Read the model definition and answer for the solid it produces. Units are mm, in the model's axes. A direction names the side the tool comes from. Give positions to 0.01 mm unless a question says otherwise; leave off trailing zeros. Order: outer loops, then holes, each group sorted by start corner. A loop starts at its lowest first (then second) coordinate and runs counter-clockwise, first axis right, second up. Notation, with made-up numbers: (71, 73) - (92, 73) arc R18 cw to (92, 96) - close; hole circle Ø4 at (27, -3). An arc over 180 degrees is marked (long way). Return JSON: item names as keys, results as strings.
Autodesk Inventor part; units mm, degrees
ref_plane "YZ Plane" through (0, 0, 0) normal (1, 0, 0) x (0, 1, 0)
ref_plane "XZ Plane" through (0, 0, 0) normal (0, 1, 0) x (-1, 0, 0)
ref_plane "XY Plane" through (0, 0, 0) normal (0, 0, 1) x (1, 0, 0)
sketch "Sketch1" plane through (0, 0, 0) normal (1, 0, 0) x (0, 1, 0)
  line L0 (0, 0) -> (241.3, 0)
  line L1 (241.3, 0) -> (241.3, -25.4)
  line L2 (241.3, -25.4) -> (0, -25.4)
  line L3 (0, -25.4) -> (0, 0)
  line L4 (6.3489, -9.0357) -> (12.6978, -5.3677)
  line L5 (12.6978, -5.3677) -> (19.0489, -9.0319)
  line L6 (19.0489, -9.0319) -> (19.0511, -16.3643)
  line L7 (19.0511, -16.3643) -> (12.7022, -20.0323)
  line L8 (12.7022, -20.0323) -> (6.3511, -16.3681)
  line L9 (6.3511, -16.3681) -> (6.3489, -9.0357)
  point P0 (12.7, -12.7)
  dimension "d0" = 241.3
  dimension "d1" = 25.4
  dimension "d3" = 12.7
  dimension "d4" = 12.7
extrude "Extrusion1" add sketch "Sketch1" along normal blind 25.4
sketch "Sketch2" plane through (0, 241.3, 0) normal (0, 1, 0) x (1, 0, 0)
  line L0 (0, 25.4) -> (25.4, 25.4)
  line L1 (0, 0) -> (25.4, 0)
  line L2 (25.4, 0) -> (25.4, 25.4)
  line L3 (25.4, 25.4) -> (0, 25.4)
  line L4 (0, 25.4) -> (0, 0)
  line L5 (22.225, 3.175) -> (3.175, 3.175)
  line L6 (3.175, 3.175) -> (3.175, 22.225)
  line L7 (3.175, 22.225) -> (22.225, 22.225)
  line L8 (22.225, 22.225) -> (22.225, 3.175)
  dimension "d7" = 3.175
extrude "Extrusion2" cut sketch "Sketch2" against normal blind 228.6 contours L5 L6 L7 L8
sketch "Sketch3" plane through (25.4, 0, 0) normal (1, 0, 0) x (0, 0, -1)
  line L0 (0, 241.3) -> (0, 190.5)
  line L1 (0, 0) -> (0, 241.3)
  line L2 (0, 241.3) -> (-3.175, 241.3)
  line L3 (-3.175, 241.3) -> (-3.175, 190.5)
  line L4 (-3.175, 190.5) -> (0, 190.5)
  line L5 (0, 190.5) -> (0, 241.3)
  arc A0 (-3.175, 241.3) -> (-46.143, 196.9282) centre (-8.4506, 203.4185) ccw
  line L6 (-3.175, 241.3) -> (-3.175, 238.125)
  arc A1 (-3.175, 238.125) -> (-42.9327, 197.9157) centre (-7.6224, 202.7623) ccw
  line L7 (-42.9327, 197.9157) -> (-46.143, 196.9282)
  dimension "d11" = 50.8
  dimension "d13" = 3.175
  dimension "d15" = 3.175
extrude "Extrusion3" add sketch "Sketch3" against normal blind 25.4 contours L0 L4 L3 L2
sketch "Sketch4" plane through (25.4, 0, 0) normal (1, 0, 0) x (0, 0, -1)
  point P0 (0, 0)
sketch "Sketch5" plane through (25.4, 0, 0) normal (1, 0, 0) x (0, 0, -1)
  line L0 (-3.175, 241.3) -> (-3.175, 190.5)
  line L1 (-3.175, 241.3) -> (-3.175, 196.85)
  line L2 (-3.175, 196.85) -> (-41.275, 196.85)
  arc A0 (-3.175, 241.3) -> (-41.275, 196.85) centre (-8.1247, 206.989) ccw
  line L3 (-41.275, 196.85) -> (-38.5091, 198.4089)
  line L4 (-3.175, 241.3) -> (-3.175, 238.125)
  arc A1 (-3.175, 238.125) -> (-38.5091, 198.4089) centre (-8.433, 207.227) ccw
  point P0 (0, 0)
  dimension "d18" = 44.45
  dimension "d19" = 38.1
  dimension "d20" = 3.175
  dimension "d21" = 3.175
extrude "Extrusion4" add sketch "Sketch5" against normal blind 25.4 contours L0 A1 L3 A0
sketch "Sketch6" plane through (25.4, 0, 0) normal (1, 0, 0) x (0, 0, -1)
  line L0 (0, 0) -> (25.4, 0)
  line L1 (25.4, 0) -> (25.4, 241.3)
  line L2 (12.7618, 20.0321) -> (19.0807, 16.3125)
  line L3 (19.0807, 16.3125) -> (19.0189, 8.9804)
  line L4 (19.0189, 8.9804) -> (12.6382, 5.3679)
  line L5 (12.6382, 5.3679) -> (6.3193, 9.0875)
  line L6 (6.3193, 9.0875) -> (6.3811, 16.4196)
  line L7 (6.3811, 16.4196) -> (12.7618, 20.0321)
  point P0 (12.7, 12.7)
  point P1 (12.7, 12.7)
  dimension "d25" = 12.7
  dimension "d26" = 12.7
  dimension "d27" = 12.7
extrude "Extrusion5" cut sketch "Sketch6" against normal blind 25.4
sketch "Sketch7" plane through (0, 0, 0) normal (-1, 0, 0) x (0, 0, 1)
  line L0 (-25.4, 241.3) -> (0, 241.3)
  line L1 (0, 241.3) -> (0, 0)
  line L2 (0, 0) -> (-25.4, 0)
  line L3 (-25.4, 0) -> (-25.4, 241.3)
extrude "Extrusion6" cut sketch "Sketch7" against normal blind 25.4
sketch "Sketch8" plane through (0, 190.5, 0) normal (0, 0, -1) x (-1, 0, 0)
  circle A0 centre (-12.7, 38.1) radius 3.175
  circle A1 centre (-12.7, 12.7) radius 3.1792
  line L0 (-25.4, 50.8) -> (0, 50.8)
  line L1 (-25.4, 0) -> (0, 0)
  point P0 (0, -190.5)
  dimension "d32" = 6.35
  dimension "d33" = 12.7
  dimension "d34" = 12.7
  dimension "d35" = 38.1
extrude "Extrusion7" cut sketch "Sketch8" against normal blind 3.175
properties part number "hand"
Q1. Consider L1, parallel to Y at x = 12.7, z = 2.3 (3 decimals); L2, parallel to Z at x = 19.25, y = 208 (3 decimals); L3, parallel to X at y = 228.6, z = 1.9 (3 decimals). Determine where each line is inside the solid, lowest interval first.
Values:
{"L1": "y = 190.5 to 200.021, 206.379 to 225.425, 231.775 to 241.3", "L2": "z = 0 to 3.175, 39.766 to 42.776", "L3": "x = 0 to 9.525, 15.875 to 25.4"}
Q2. A cutting plane is placed at C-C (y = 228.6). Write down the section's boundary in (x, z) (3 decimals).
Values:
{"outline": "(0, 0) - (9.525, 0) - (9.525, 3.175) - (0, 3.175) - close; (0, 31.357) - (25.4, 31.357) - (25.4, 35.23) - (0, 35.23) - close; (15.875, 0) - (25.4, 0) - (25.4, 3.175) - (15.875, 3.175) - close"}
Q3. A cutting plane is placed at B-B (y = 217). Write down the section's boundary in (x, z) (3 decimals).
Values:
{"outline": "(0, 0) - (25.4, 0) - (25.4, 3.175) - (0, 3.175) - close; (0, 38.213) - (25.4, 38.213) - (25.4, 41.314) - (0, 41.314) - close"}
Q4. Determine the mould class of faces 4 (the flat face through (0, 224, 2)), 5 (the cylindrical face through (13.39, 225.5, 1.57)), 6 (the flat face through (13, 215, 3.175)) for opening direction X: released by +X, released by -X, zero draft, split by the parting line, or undercut.
Values:
{"face 4": "released by -X", "face 5": "undercut", "face 6": "zero draft"}
Q5. A cutting plane is placed at D-D (x = 17.75). Write down the section's boundary in (y, z) (3 decimals), and give its area (3 significant figures).
Values:
{"outline": "(190.5, 0) - (241.3, 0) - (241.3, 3.175) arc R34.666 ccw to (196.85, 41.275) - (198.409, 38.509) arc R31.342 cw to (238.125, 3.175) - (190.5, 3.175) - close", "area": "361 mm²"}
Q6. Given pin 1 (1 mm diameter, centred on x = 8, z = 7.5, fed in from +Y); pin 2 (6 mm diameter, centred on x = 16, z = 21, fed in from -Y); pin 3 (5 mm diameter, centred on x = 18.5, z = 23, fed in from -Y), each flat-ended and moving along its own axis, determine where each tip first touches the part or whether it passes through.
Values:
{"pin 1": "stops at y = 241.65", "pin 2": "stops at y = 234.43", "pin 3": "stops at y = 233.51"}
Q7. A cutting plane is placed at A-A (x = 12.7). Write down the section's boundary in (y, z) (3 decimals), and give its area (3 significant figures).
Values:
{"outline": "(190.5, 0) - (200.021, 0) - (200.021, 3.175) - (190.5, 3.175) - close; (196.85, 41.275) - (198.409, 38.509) arc R31.342 cw to (238.125, 3.175) - (231.775, 3.175) - (231.775, 0) - (241.3, 0) - (241.3, 3.175) arc R34.666 ccw to start; (206.379, 0) - (225.425, 0) - (225.425, 3.175) - (206.379, 3.175) - close", "area": "321 mm²"}
Q8. For faces 1 (the cylindrical face through (15.223, 201.266, 1.565)), 2 (the flat face through (13, 241.3, 2)), 3 (the flat face through (12.88, 197.62, 39.91)), determine the directions among +Z, -Z, +X, -X, +Y, -Y from which every point of the face is accessible in a straight line to the end or side of a thin tool.
Values:
{"face 1": "-Z", "face 2": "-Z, +X, -X, +Y", "face 3": "+X, -X, -Y"}
